Input: dimensioned drawing with shaded views. Units: mm. Origin: part minimum x, y, z. A direction names the side the tool comes from. Coordinates: 2 decimals unless noted, no trailing zeros. Order: outer loops, then holes, each group sorted by start corner. A loop starts at its lowest first (then second) coordinate and runs counter-clockwise, first axis right, second up. Notation, with made-up numbers: (87, 5) -> (91, 5) arc R15 ccw to (91, 14) -> close; hole circle Ø7 at (85, 68). An arc over 180 degrees is marked (long way). Answer as CSV lines item,"result".
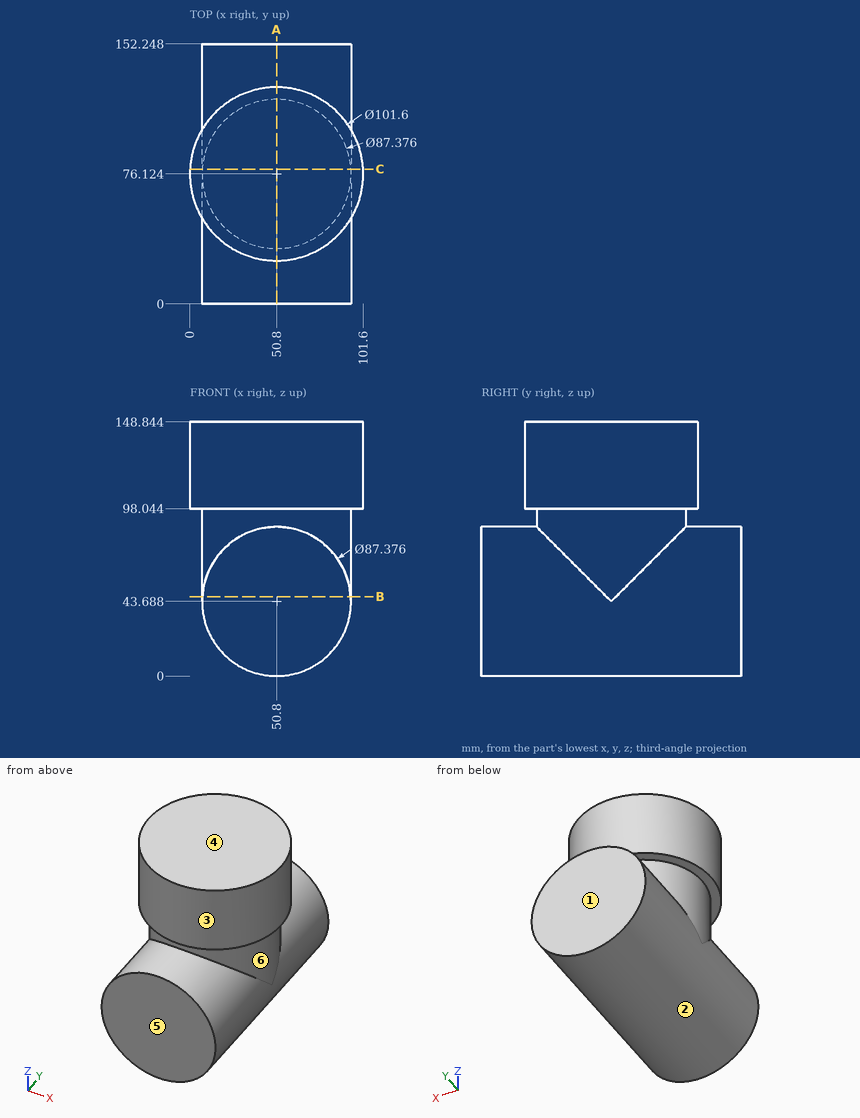
1. Cut plane C-C (y = 79). Return the cut outline in (x, z) (1 decimal), plus the area to 3 significant figures.
Findings:
outline,"(0.1, 98) -> (7.2, 98) -> (7.2, 46.6) arc R43.7 ccw (long way) to (94.4, 46.6) -> (94.4, 98) -> (101.5, 98) -> (101.5, 148.8) -> (0.1, 148.8) -> close"
area,"12,900 mm2"
2. Ray query, line 1 along X through (y, z) = (102, 129) (1 decimal); line 2 along X through (y, z) = (16, 26.5) (1 decimal); line 3 along Y through (x, z) = (81, 85) (1 decimal). Return the intervals inside material, ascending.
Findings:
line 1,"x = 7.1 to 94.5"
line 2,"x = 10.6 to 91"
line 3,"y = 44.6 to 107.7"
3. Reachability of the marked faces 1, 2 and 3 from +Z, -Z, +X, -X, +Y, -Y: full face, straight path, thin tool, end or side. Return the list, or none.
Findings:
face 1,"+Z, -Z, +X, -X, +Y"
face 2,"none"
face 3,"+Z"
4. Contact query for flat-ended pins moving along their axis: pin 1 (10 mm diameter, centred on x = 46.5, y = 77, fed in from -Z); pin 2 (4 mm diameter, centred on y = 41, z = 70, fed in from -X); pin 3 (8 mm diameter, centred on x = 25, z = 129.5, fed in from -Y). Output: stop coordinate, or through.
Findings:
pin 1,"stops at z = 0"
pin 2,"stops at x = 14.5"
pin 3,"stops at y = 30.24"
5. Cut plane B-B (z = 46.5). Return the cut outline in (x, y) (1 decimal).
Findings:
outline,"(7.2, 0) -> (94.4, 0) -> (94.4, 73.3) arc R43.7 ccw to (94.4, 78.9) -> (94.4, 152.2) -> (7.2, 152.2) -> (7.2, 78.9) arc R43.7 ccw to (7.2, 73.3) -> close"
6. Mould query, pull axis Z, two halves, no side actions, for the marked faces 4, 5 and 6. Classes: released by +Z, released by -Z, zero draft, split by the parting line, or undercut.
Findings:
face 4,"released by +Z"
face 5,"zero draft"
face 6,"undercut"
7. Cut plane A-A (x = 50.8). Return the cut outline in (y, z) (1 decimal).
Findings:
outline,"(0, 0) -> (152.2, 0) -> (152.2, 87.4) -> (119.8, 87.4) -> (119.8, 98) -> (126.9, 98) -> (126.9, 148.8) -> (25.3, 148.8) -> (25.3, 98) -> (32.4, 98) -> (32.4, 87.4) -> (0, 87.4) -> close"
